```python
from build123d import *

# Parameters (mm, degrees)
SKETCH_W        = 65
SKETCH_H        = 56
SKETCH_R        = 1.45
PAD_DEPTH       = 4
SKETCH002_R     = 1.25
POCKET_DEPTH    = 5
SKETCH005_W     = 19
SKETCH005_H     = 4
PAD002_DEPTH    = 50
SKETCH006_W     = 8
SKETCH006_H     = 4
PAD003_DEPTH    = 5
SKETCH007_W     = 8
SKETCH007_H     = 4
PAD004_DEPTH    = 4
PAD004_FACE36_W = 8
PAD004_FACE36_H = 4
PAD005_DEPTH    = 8
SKETCH008_R     = 1.75
POCKET001_DEPTH = 4.001
CHAMFER_SIZE    = 1


with BuildPart() as part:
    # Sketch → Pad (new body)
    with BuildSketch(Plane.XY):
        with Locations((32.5, 28)):
            Rectangle(SKETCH_W, SKETCH_H)
        with Locations((3.5, 52.5)):
            Circle(SKETCH_R, mode=Mode.SUBTRACT)
        with Locations((61.5, 52.5)):
            Circle(SKETCH_R, mode=Mode.SUBTRACT)
        with Locations((3.5, 3.5)):
            Circle(SKETCH_R, mode=Mode.SUBTRACT)
        with Locations((61.5, 3.5)):
            Circle(SKETCH_R, mode=Mode.SUBTRACT)
        Polygon((7.782759, 51.5), (57.217241, 51.5), (32.5, 30.618193), align=None, mode=Mode.SUBTRACT)
        Polygon((60.5, 49.036979), (60.5, 6.963021), (35.599086, 28), align=None, mode=Mode.SUBTRACT)
        Polygon((57.217241, 4.5), (7.782759, 4.5), (32.5, 25.381807), align=None, mode=Mode.SUBTRACT)
        Polygon((4.5, 6.963021), (4.5, 49.036979), (29.400914, 28), align=None, mode=Mode.SUBTRACT)
    extrude(amount=PAD_DEPTH)

    # Sketch002 → Pocket (cut)
    with BuildSketch(Plane(origin=(-1.55844, 1.844684, 0), x_dir=(-0.763886, -0.645352, 0), z_dir=(-0.645352, 0.763886, 0))):
        with Locations((-21.5, 5.25)):
            Circle(SKETCH002_R)
        with Locations((-4.5, 5.25)):
            Circle(SKETCH002_R)
    extrude(amount=-POCKET_DEPTH, mode=Mode.SUBTRACT)

    # Sketch005 → Pad002 (join)
    with BuildSketch(Plane.YZ.offset(65)):
        with Locations((9.5, 2)):
            Rectangle(SKETCH005_W, SKETCH005_H)
    extrude(amount=PAD002_DEPTH)

    # Sketch006 (on Face1 of Pad002) → Pad003 (join)
    with BuildSketch(Plane(origin=(0, 56, 0), x_dir=(-1, 0, 0), z_dir=(0, 1, 0))):
        with Locations((-11, 2)):
            Rectangle(SKETCH006_W, SKETCH006_H)
    extrude(amount=PAD003_DEPTH)

    # Sketch007 (on Face6 of Pad003) → Pad004 (join)
    with BuildSketch(Plane(origin=(0, 0, 0), x_dir=(1, 0, 0), z_dir=(0, 0, -1))):
        with Locations((11, -59)):
            Rectangle(SKETCH007_W, SKETCH007_H)
    extrude(amount=PAD004_DEPTH)

    # Pad004 Face36 → Pad005 (add)
    with BuildSketch(Plane(origin=(11, 61, -2), x_dir=(1, 0, 0), z_dir=(0, 1, 0))):
        Rectangle(PAD004_FACE36_W, PAD004_FACE36_H)
    extrude(amount=PAD005_DEPTH)

    # Sketch008 (on Face9 of Pad005) → Pocket001 (cut, through all)
    with BuildSketch(Plane(origin=(0, 0, 0), x_dir=(1, 0, 0), z_dir=(0, 0, -1))):
        with Locations((105, -3)):
            Circle(SKETCH008_R)
        with Locations((100.5, -14)):
            Circle(SKETCH008_R)
    extrude(amount=-POCKET001_DEPTH, mode=Mode.SUBTRACT)

    # Chamfer
    chamfer_edges = [part.edges().sort_by_distance(p)[0] for p in [
        (98.75, 14, 0),
        (103.25, 3, 0),
    ]]
    chamfer(chamfer_edges, length=CHAMFER_SIZE)


solid = part.part
```
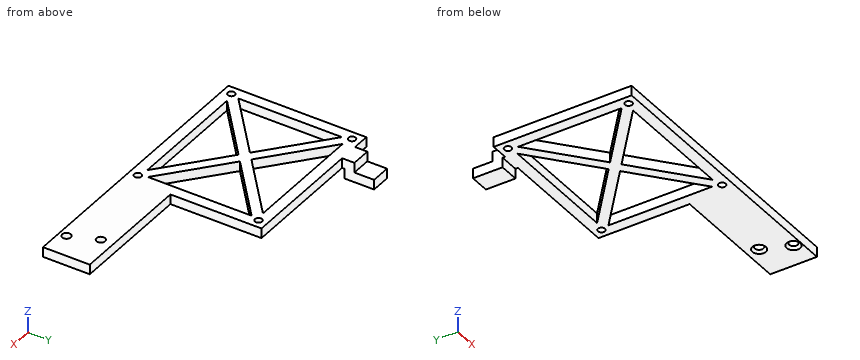
Verification items for the finished model (mm, model axes). Round coordinates to 2 decimals unless told otherwise and drop trailing zeros. Order: outer loops, then holes, each group sorted by start corner. A loop starts at its lowest first (then second) coordinate and runs counter-clockwise, first axis right, second up.
1) Cross-section at C-C, the plane y = 14. Record the cut outline in (x, z).
Geometry says:
outline: (0, 0) - (4.5, 0) - (4.5, 4) - (0, 4) - close; (12.83, 0) - (19.03, 0) - (19.03, 4) - (12.83, 4) - close; (45.97, 0) - (52.17, 0) - (52.17, 4) - (45.97, 4) - close; (60.5, 0) - (97.75, 0) - (98.75, 1) - (98.75, 4) - (60.5, 4) - close; (102.25, 1) - (103.25, 0) - (115, 0) - (115, 4) - (102.25, 4) - close
2) Cross-section at A-A, the plane x = 105. Record the cut outline in (y, z).
Geometry says:
outline: (0, 0) - (0.25, 0) - (1.25, 1) - (1.25, 4) - (0, 4) - close; (4.75, 1) - (5.75, 0) - (19, 0) - (19, 4) - (4.75, 4) - close
3) Cross-section at D-D, the plane x = 44. Record the cut outline in (y, z).
Geometry says:
outline: (0, 0) - (4.5, 0) - (4.5, 4) - (0, 4) - close; (15.67, 0) - (20.9, 0) - (20.9, 4) - (15.67, 4) - close; (35.1, 0) - (40.33, 0) - (40.33, 4) - (35.1, 4) - close; (51.5, 0) - (56, 0) - (56, 4) - (51.5, 4) - close
4) Cross-section at B-B, the plane y = 38. Record the cut outline in (x, z).
Geometry says:
outline: (0, 0) - (4.5, 0) - (4.5, 4) - (0, 4) - close; (17.56, 0) - (23.76, 0) - (23.76, 4) - (17.56, 4) - close; (41.24, 0) - (47.44, 0) - (47.44, 4) - (41.24, 4) - close; (60.5, 0) - (65, 0) - (65, 4) - (60.5, 4) - close
5) Depth check by flat-ended pin: pin 1 (1.2 mm diameter, centred on y = 31, z = 2.5, fed in from -X); pin 2 (2 mm diameter, centred on x = 33.5, z = 2, fed in from +Y); pin 3 (1.2 mm diameter, centred on x = 9.5, z = -2.5, fed in from -Y); pin 4 (3 mm diameter, centred on x = 105, y = 3, fed in from -Z). Enter the tip coordinate at first touch or a pass-through.
Geometry says:
pin 1: stops at x = 0
pin 2: stops at y = 56
pin 3: stops at y = 57
pin 4: passes through
6) Material ranges on line 1 (Y direction, x = 61.5, z = 2.3); line 2 (X direction, y = 34.5, z = 2.25); line 3 (X direction, y = 48, z = 0.75), recorded low to high.
Geometry says:
line 1: y = 0 to 2.05, 4.95 to 51.05, 53.95 to 56
line 2: x = 0 to 4.5, 21.71 to 27.91, 37.09 to 43.29, 60.5 to 65
line 3: x = 0 to 4.5, 5.73 to 11.93, 53.07 to 59.27, 60.5 to 65
